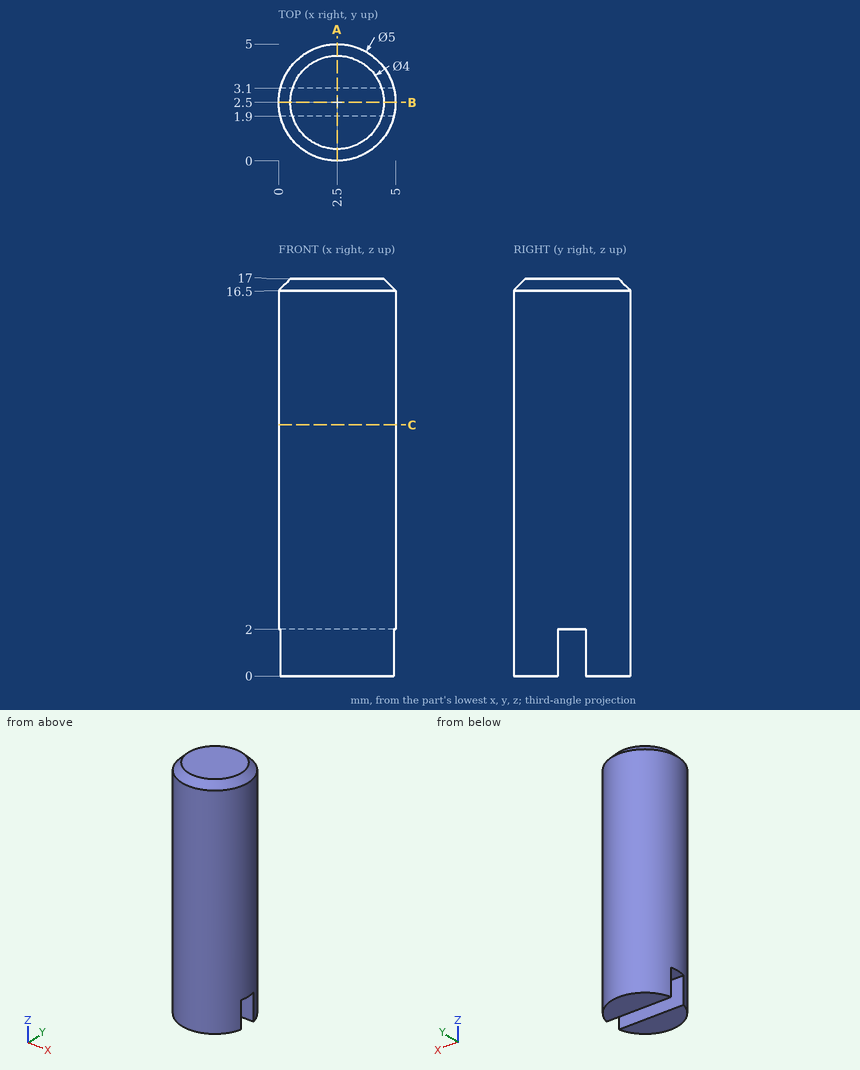
Job drawing, mm, ordinate dimensions from the low corner. One solid piece. Coordinates: 2 decimals unless noted, no trailing zeros. Write each loop counter-clockwise with the first axis right and the second up, starting at its lowest first coordinate (ties: lowest second). Pieces come first, ordered by that corner, then holes. Notation, with made-up numbers: (23.5, 17) - (44.5, 17) arc R25 cw to (44.5, 34) - close; hole circle Ø4 at (70, 86.25). An arc over 180 degrees is marked (long way). Use a Markdown table: item, result. Add a question column.
Item 1: Band-saw the part on A-A, the plane x = 2.5. Give the cut face in (y, z), and give its area (4 significant figures).
Item 2: Flat gauge pin, fed straight in: pin 1 (2 mm diameter, centred on y = 0.5, z = 9, fed in from +X). Where does the tip first touch, or does it go through?
Item 3: Drill centre lines: L1, parallel to Y at x = 1.9, z = 8.5; L2, parallel to X at y = 4, z = 13; L3, parallel to Y at x = 1.85, z = 1. Where is each one in solid material? Low to high. Write a range as from..to.
Item 4: Band-saw the part on B-B, the plane y = 2.5. Give the cut face in (x, z).
Item 5: Band-saw the part on C-C, the plane z = 10.75. Give the cut face in (x, y).
Numbers:
| question | item | result |
|---|---|---|
| 1 | outline | (0, 0) - (1.9, 0) - (1.9, 2) - (3.1, 2) - (3.1, 0) - (5, 0) - (5, 16.5) - (4.5, 17) - (0.5, 17) - (0, 16.5) - close |
| 1 | area | 82.35 mm2 |
| 2 | pin 1 | x = 4.79 |
| 3 | L1 | 0.07..4.93 |
| 3 | L2 | 0.5..4.5 |
| 3 | L3 | 0.09..1.9, 3.1..4.91 |
| 4 | outline | (0, 2) - (5, 2) - (5, 16.5) - (4.5, 17) - (0.5, 17) - (0, 16.5) - close |
| 5 | outline | circle Ø5 at (2.5, 2.5) |
